```python
from build123d import *

# Parameters (mm, degrees)
SKETCH1_W             = 25
SKETCH1_H             = 25
BOSS_EXTRUDE1_DEPTH   = 250
BOSS_EXTRUDE1_2_DEPTH = 250
SKETCH2_R             = 5.3
CUT_EXTRUDE1_DEPTH    = 263.183618863
BOSS_EXTRUDE2_REACH   = 264.184
SKETCH4_W             = 25
SKETCH4_H             = 28
CUT_EXTRUDE2_DEPTH    = 254.332291665
BOSS_EXTRUDE3_START   = -53
SKETCH5_R             = 5
BOSS_EXTRUDE3_DEPTH   = 28
SKETCH6_W             = 25
SKETCH6_H             = 130
BOSS_EXTRUDE4_DEPTH   = 25
SKETCH7_W             = 25
SKETCH7_H             = 28
CUT_EXTRUDE3_DEPTH    = 323


with BuildPart() as part:
    # Sketch1 → Boss-Extrude1 (new body)
    with BuildSketch(Plane(origin=(0, 0, 0), x_dir=(1, 0, 0), z_dir=(0, 1, 0))):
        with Locations((0, 26.5)):
            Rectangle(SKETCH1_W, SKETCH1_H)
    extrude(amount=BOSS_EXTRUDE1_DEPTH)


with BuildPart() as body_2:
    # Sketch1 → Boss-Extrude1 2 (new body)
    with BuildSketch(Plane(origin=(0, 0, 0), x_dir=(1, 0, 0), z_dir=(0, 1, 0))):
        with Locations((0, -26.5)):
            Rectangle(SKETCH1_W, SKETCH1_H)
    extrude(amount=BOSS_EXTRUDE1_2_DEPTH)


with BuildPart() as cut_extrude1_tool:
    # Sketch2 → Cut-Extrude1 (new, through all)
    with BuildSketch(Plane.XY.offset(39)):
        with Locations((0, 237.5)):
            Circle(SKETCH2_R)
    extrude(amount=-CUT_EXTRUDE1_DEPTH)


with BuildPart() as part_1:
    add(part.part)

    # Cut-Extrude1: cut by cut_extrude1_tool
    add(cut_extrude1_tool.part, mode=Mode.SUBTRACT)

    # Boss-Extrude2: up to this face of the body (flat: up to its plane)
    boss_extrude2_end = Plane(part_1.part.faces().sort_by_distance((0, 123.388798443, -39))[0])
    # Sketch3 → Boss-Extrude2 (add, up to the picked face)
    with BuildSketch(Plane.XY.offset(39), mode=Mode.PRIVATE) as boss_extrude2_sk1:
        with BuildLine():
            Line((-12.5, 250), (-4.8, 276.4))
            ThreePointArc((-4.8, 276.4), (0, 280), (4.8, 276.4))
            Line((4.8, 276.4), (12.5, 250))
            Line((12.5, 250), (-12.5, 250))
        make_face()
    boss_extrude2_tool1 = split(extrude(boss_extrude2_sk1.sketch, amount=-BOSS_EXTRUDE2_REACH, mode=Mode.PRIVATE), bisect_by=boss_extrude2_end, keep=Keep.BOTH, mode=Mode.PRIVATE)


with BuildPart() as body_2_1:
    add(body_2.part)

    # Cut-Extrude1: cut by cut_extrude1_tool
    add(cut_extrude1_tool.part, mode=Mode.SUBTRACT)


with BuildPart() as part_2:
    add(part_1.part)

    add(body_2_1.part)  # Boss-Extrude2 merges body 2
    add(boss_extrude2_tool1.solids().sort_by(Axis((0, 262.12086, 39), (0, 0, -1)))[0])

    # Sketch4 → Cut-Extrude2 (cut, through all)
    with BuildSketch(Plane.XZ.offset(-250)):
        Rectangle(SKETCH4_W, SKETCH4_H)
    extrude(amount=-CUT_EXTRUDE2_DEPTH, mode=Mode.SUBTRACT)


with BuildPart() as cut_extrude2_piece_1:
    # of the separate pieces the step leaves, piece 1, a body of its own (cut_extrude2_pieces)
    add(part_2.part.solids().sort_by_distance((4.8, 276.4, 39))[0])



with BuildPart() as cut_extrude2_piece_2:
    # of the separate pieces the step leaves, piece 2, a body of its own (cut_extrude2_pieces)
    add(part_2.part.solids().sort_by_distance((12.5, 250, -14))[0])


with BuildPart() as cut_extrude2_piece_1_1:
    add(cut_extrude2_piece_1.part)

    add(cut_extrude2_piece_2.part)  # Boss-Extrude3 merges Cut-Extrude2 piece 2
    # Sketch5 → Boss-Extrude3 (add)
    with BuildSketch(Plane(origin=(0, 0, -39), x_dir=(-1, 0, 0), z_dir=(0, 0, -1)).offset(BOSS_EXTRUDE3_START)):
        with Locations(Location((0, 275, 0), (0, 0, 163.739795292))):
            Circle(SKETCH5_R)
    extrude(amount=BOSS_EXTRUDE3_DEPTH)

    # Sketch6 → Boss-Extrude4 (add)
    with BuildSketch(Plane.XZ):
        Rectangle(SKETCH6_W, SKETCH6_H)
    extrude(amount=BOSS_EXTRUDE4_DEPTH)

    # Sketch7 → Cut-Extrude3 (cut)
    with BuildSketch(Plane(origin=(0, 0, 0), x_dir=(1, 0, 0), z_dir=(0, 1, 0))):
        Rectangle(SKETCH7_W, SKETCH7_H)
    extrude(amount=CUT_EXTRUDE3_DEPTH, mode=Mode.SUBTRACT)


solid = cut_extrude2_piece_1_1.part
```
The listing builds one solid part. Answer for the finished solid, in the listing's coordinates (mm). A direction names the side the tool comes from. Give positions to 0.01 mm unless a question says otherwise; leave off trailing zeros. Order: outer loops, then holes, each group sorted by start corner. A loop starts at its lowest first (then second) coordinate and runs counter-clockwise, first axis right, second up. Notation, with made-up numbers: (39.5, 56.5) - (96.5, 56.5) arc R22 ccw to (96.5, 90.5) - close; hole circle Ø7 at (-38.75, -20.75). An arc over 180 degrees is marked (long way). Use one line per item in the form item = value. Start each with the question number.
(1) For faces 1 (the flat face through (0, 142, 39)), 2 (the flat face through (-12.5, 84, -15)), 3 (the flat face through (0, 138, -14)), 4 (the flat face through (0, 138, -39)), determine the directions among +Z, -Z, +X, -X, +Y, -Y from which every point of the face is accessible in a straight line to the end or side of a thin tool.
(2) A cutting plane is placed at C-C, the plane y = 149. Write down the section's boundary in (x, z).
(3) A cutting plane is placed at D-D, the plane y = 237.5. Write down the section's boundary in (x, z), then the cut area to 3 significant figures.
(4) A cutting plane is placed at B-B, the plane z = 18. Write down the section's boundary in (x, y), then the cut area to 3 significant figures.
(5) Flat-ended cylindrical pins translate along their axes: pin 1 Ø12.5 at (x, z) = (-0.5, -50) entering from +Y; pin 2 Ø5 at (x, y) = (5, 61) entering from +Z; pin 3 Ø12.5 at (x, y) = (-2, 96) entering from -Z. Find the tip coordinate at first contact, or state that the pin passes through.
(6) The mould has two halves that part along X. Classify faces 5 (the cylindrical face through (-0.69, 242.755, -26.325)), 6 (the flat face through (-8.704, 263.015, -26.325)), 7 (the flat face through (0, 0, -52)): released by +X, released by -X, zero draft, split by the parting line, or undercut.
(7) A cutting plane is placed at A-A, the plane x = 0. Write down the section's boundary in (y, z), then the cut area to 3 significant figures.
(8) Consider line 1 (Y direction, x = 0, z = 21.75); line 2 (Z direction, x = 4, y = 245); line 3 (Y direction, x = -7.25, z = -3). Determine where each line is inside the solid, lowest interval first. Write a range as from..to.
Ans:
q1.face_1 = +Z, +X, -X, +Y
q1.face_2 = +Z, -Z, -X, +Y, -Y
q1.face_3 = +X, -X, +Y
q1.face_4 = -Z, +X, -X, +Y
q2.outline = (-12.5, -39) - (12.5, -39) - (12.5, -14) - (-12.5, -14) - close; (-12.5, 14) - (12.5, 14) - (12.5, 39) - (-12.5, 39) - close
q3.outline = (-12.5, -39) - (-5.3, -39) - (-5.3, -14) - (-12.5, -14) - close; (-12.5, 14) - (-5.3, 14) - (-5.3, 39) - (-12.5, 39) - close; (5.3, -39) - (12.5, -39) - (12.5, -14) - (5.3, -14) - close; (5.3, 14) - (12.5, 14) - (12.5, 39) - (5.3, 39) - close
q3.area = 720 mm^2
q4.outline = (-12.5, -25) - (12.5, -25) - (12.5, 250) - (4.8, 276.4) arc R5 ccw to (-4.8, 276.4) - (-12.5, 250) - close; hole circle Ø10.6 at (0, 237.5)
q4.area = 7,270 mm^2
q5.pin_1 = 0
q5.pin_2 = 39
q5.pin_3 = -39
q6.face_5 = undercut
q6.face_6 = released by -X
q6.face_7 = zero draft
q7.outline = (-25, -65) - (0, -65) - (0, -39) - (232.2, -39) - (232.2, -14) - (0, -14) - (0, 14) - (232.2, 14) - (232.2, 39) - (0, 39) - (0, 65) - (-25, 65) - close; (242.8, -39) - (280, -39) - (280, -14) - (242.8, -14) - close; (242.8, 14) - (280, 14) - (280, 39) - (242.8, 39) - close
q7.area = 16,700 mm^2
q8.line_1 = -25..232.2, 242.8..280
q8.line_2 = -39..-14, 14..39
q8.line_3 = -25..0
